Read the model definition and answer for the solid it produces. Units are mm, in the model's axes. Face numbers are marked on the shaded views. A direction names the side the tool comes from. Coordinates: 2 decimals unless noted, no trailing zeros. Order: outer loops, then holes, each group sorted by start corner. A loop starts at its lowest first (then second) coordinate and runs counter-clockwise, first axis right, second up. Notation, with made-up numbers: (79, 40.5) - (121, 40.5) arc R14 cw to (121, 54.5) - close; hole circle Ø8 at (-4, 19.5). An arc over 180 degrees is marked (long way). Answer as a JSON object with one key per item and string values. Group by question number.
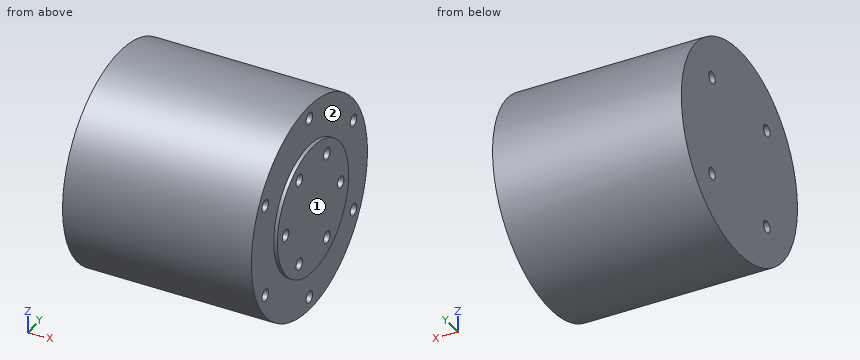
from build123d import *

# Parameters (mm, degrees)
SKETCH_1_R          = 28.5
EXTRUDE_1_DEPTH     = 51
SKETCH_2_R          = 17.5
EXTRUDE_2_DEPTH     = 1
SKETCH_3_R          = 1.6
CUT_EXTRUDE_1_DEPTH = 5
SKETCH_4_R          = 1.6
CUT_EXTRUDE_2_DEPTH = 5
SKETCH_5_R          = 1.6
CUT_EXTRUDE_3_DEPTH = 5


with BuildPart() as part:
    # 草图1 → 凸台-拉伸1 (new body)
    with BuildSketch(Plane(origin=(0, 0, 0), x_dir=(0, 0, -1), z_dir=(1, 0, 0))):
        Circle(SKETCH_1_R)
    extrude(amount=EXTRUDE_1_DEPTH)

    # 草图2 → 凸台-拉伸2 (add)
    with BuildSketch(Plane(origin=(51, 0, 0), x_dir=(0, 0, -1), z_dir=(1, 0, 0))):
        Circle(SKETCH_2_R)
    extrude(amount=EXTRUDE_2_DEPTH)

    # 草图3 → 切除-拉伸1 (cut)
    with BuildSketch(Plane.ZY):
        with Locations((13.435028843, 13.435028843)):
            Circle(SKETCH_3_R)
        with Locations((13.435028843, -13.435028843)):
            Circle(SKETCH_3_R)
        with Locations((-13.435028843, -13.435028843)):
            Circle(SKETCH_3_R)
        with Locations((-13.435028843, 13.435028843)):
            Circle(SKETCH_3_R)
    extrude(amount=-CUT_EXTRUDE_1_DEPTH, mode=Mode.SUBTRACT)

    # 草图4 → 切除-拉伸2 (cut)
    with BuildSketch(Plane(origin=(51, 0, 0), x_dir=(0, 0, -1), z_dir=(1, 0, 0))):
        with Locations((-12.5, 21.650635095)):
            Circle(SKETCH_4_R)
        with Locations((12.5, 21.650635095)):
            Circle(SKETCH_4_R)
        with Locations((25, 0)):
            Circle(SKETCH_4_R)
        with Locations((12.5, -21.650635095)):
            Circle(SKETCH_4_R)
        with Locations((-12.5, -21.650635095)):
            Circle(SKETCH_4_R)
        with Locations((-25, 0)):
            Circle(SKETCH_4_R)
    extrude(amount=-CUT_EXTRUDE_2_DEPTH, mode=Mode.SUBTRACT)

    # 草图5 → 切除-拉伸3 (cut)
    with BuildSketch(Plane(origin=(52, 0, 0), x_dir=(0, 0, -1), z_dir=(1, 0, 0))):
        with Locations((0, 13.5)):
            Circle(SKETCH_5_R)
        with Locations((11.691342951, 6.75)):
            Circle(SKETCH_5_R)
        with Locations((11.691342951, -6.75)):
            Circle(SKETCH_5_R)
        with Locations((0, -13.5)):
            Circle(SKETCH_5_R)
        with Locations((-11.691342951, -6.75)):
            Circle(SKETCH_5_R)
        with Locations((-11.691342951, 6.75)):
            Circle(SKETCH_5_R)
    extrude(amount=-CUT_EXTRUDE_3_DEPTH, mode=Mode.SUBTRACT)


solid = part.part
1. Given pin 1 (4 mm diameter, centred on x = 29.5, z = 6.5, fed in from +Y); pin 2 (2.5 mm diameter, centred on y = 13.44, z = 13.44, fed in from -X); pin 3 (1.5 mm diameter, centred on x = 21, z = 3, fed in from +Y), each flat-ended and moving along its own axis, determine where each tip first touches the part or whether it passes through.
2. A cutting plane is placed at C-C on x = 11. Write down the section's boundary in (y, z), and give its area (3 significant figures).
3. A cutting plane is placed at B-B on y = 0. Write down the section's boundary in (x, z).
4. A cutting plane is placed at D-D on y = -11. Write down the section's boundary in (x, z), and give its area (3 significant figures).
5. Straight lines are drawn through the part: L1, parallel to Y at x = 48, z = -12.5; L2, parallel to X at y = 10, z = 18; L3, parallel to Z at x = 49, y = -6. For each, find the intervals that lie inside material, in ascending order.
6. For the marked faces 1 and 2, determine the directions among +Z, -Z, +X, -X, +Y, -Y from which every point of the face is accessible in a straight line to the end or side of a thin tool.
7. A cutting plane is placed at A-A on z = 0. Write down the section's boundary in (x, y), and give its area (3 significant figures).
Derived:
{
 "1": {"pin 1": "stops at y = 28.14", "pin 2": "stops at x = 5", "pin 3": "stops at y = 28.41"},
 "2": {"outline": "circle Ø57 at (0, 0)", "area": "2,550 mm2"},
 "3": {"outline": "(0, -28.5) - (51, -28.5) - (51, -26.6) - (46, -26.6) - (46, -23.4) - (51, -23.4) - (51, -17.5) - (52, -17.5) - (52, 17.5) - (51, 17.5) - (51, 23.4) - (46, 23.4) - (46, 26.6) - (51, 26.6) - (51, 28.5) - (0, 28.5) - close"},
 "4": {"outline": "(0, -26.29) - (51, -26.29) - (51, -13.61) - (52, -13.61) - (52, 13.61) - (51, 13.61) - (51, 26.29) - (0, 26.29) - close", "area": "2,710 mm2"},
 "5": {"L1": "y = -25.61 to -23.25, -20.05 to -8.13, -5.37 to 5.37, 8.13 to 20.05, 23.25 to 25.61", "L2": "x = 0 to 51", "L3": "z = -27.86 to -13.1, -10.28 to 10.28, 13.1 to 27.86"},
 "6": {"face 1": "+Z, -Z, +X, +Y, -Y", "face 2": "+X"},
 "7": {"outline": "(0, -28.5) - (51, -28.5) - (51, -17.5) - (52, -17.5) - (52, -15.1) - (47, -15.1) - (47, -11.9) - (52, -11.9) - (52, 11.9) - (47, 11.9) - (47, 15.1) - (52, 15.1) - (52, 17.5) - (51, 17.5) - (51, 28.5) - (0, 28.5) - close", "area": "2,910 mm2"}
}
